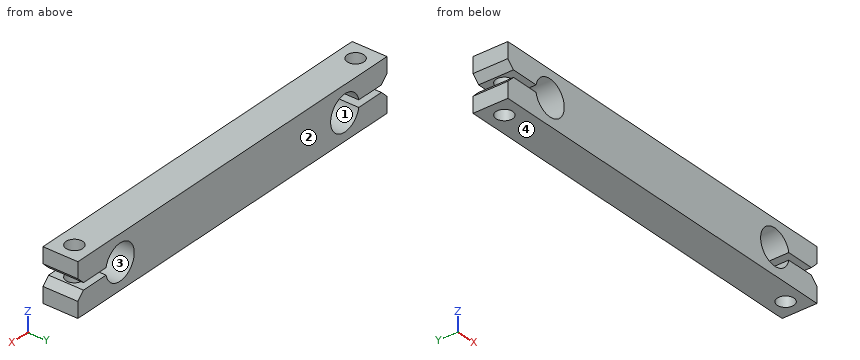
```python
from build123d import *

# Parameters (mm, degrees)
F0_W     = 34.925
F0_H     = 9.525
F0_R     = 3.2131
F1_DEPTH = 6.35
F2_R     = 1.524
F3_DEPTH = 9.525
F5_DEPTH = 6.351
F6_SIZE  = 1.27


with BuildPart() as f1:
    # F0 (on Front) → F1 (new body)
    with BuildSketch(Plane.XZ):
        with Locations((17.4625, 0)):
            Rectangle(F0_W, F0_H)
        with Locations((25.4, 0)):
            Circle(F0_R, mode=Mode.SUBTRACT)
    extrude(amount=F1_DEPTH)

    # F2 (on face) → F3 (cut, through all)
    with BuildSketch(Plane.XY.offset(4.7625)):
        with Locations((31.76905, -3.175)):
            Circle(F2_R)
    extrude(amount=-F3_DEPTH, mode=Mode.SUBTRACT)

    # F4 (on face) → F5 (cut, through all)
    with BuildSketch(Plane(origin=(0, 0, 0), x_dir=(-1, 0, 0), z_dir=(0, 1, 0))):
        with BuildLine():
            Line((-28.5497280216, 0.635), (-34.925, 0.635))
            Line((-34.925, 0.635), (-34.925, -0.635))
            Line((-34.925, -0.635), (-28.5497280216, -0.635))
            ThreePointArc((-28.5497280216, -0.635), (-28.6131, 0), (-28.5497280216, 0.635))
        make_face()
    extrude(amount=-F5_DEPTH, mode=Mode.SUBTRACT)

    # F6
    f6_edges = [f1.edges().sort_by_distance(p)[0] for p in [
        (34.925, -3.175, 0.635),
        (34.925, -3.175, -0.635),
    ]]
    chamfer(f6_edges, length=F6_SIZE)

    # F7: F1 across face


with BuildPart() as f1_1:
    add(f1.part)
    add(f1.part.mirror(Plane(origin=(0, -3.175, 0), x_dir=(0, -1, 0), z_dir=(-1, 0, 0))))


solid = f1_1.part
```
Build history of the part. All positions in model axes, mm. Face numbers are marked on the shaded views. Give positions to 0.01 mm unless a question says otherwise; leave off trailing zeros. Order: outer loops, then holes, each group sorted by start corner. A loop starts at its lowest first (then second) coordinate and runs counter-clockwise, first axis right, second up. Notation, with made-up numbers: M 56.25,69.25 L 81.25,69.25 A24 ccw 81.25,85.25 Z; hole C 68.5,-18.5 d10. An arc over 180 degrees is marked long. Write item = value, one per line. Start each with the question number.
(1) Two-plate mould, pull along Z, no slides. Class the marked faces 1, 2, 3 and 4: released by +Z, released by -Z, zero draft, split by the parting line, or undercut.
(2) Pin check, flat tip, straight feed: pin 1 Ø1.8 at (x, y) = (31.77, -3.18) entering from -Z. Stop position of the tip, or through.
(3) Slice it at A-A on x = -25.4. Write the cut outline in (y, z).
(4) Slice it at D-D on z = 0. Write the cut outline in (x, y), plus the area to 3 significant figures.
(5) Slice it at C-C on y = -0.75. Write the cut outline in (x, z) (1 decimal).
(6) Slice it at B-B on z = 2.5. Write the cut outline in (x, y) (3 decimals).
(7) Probe L1, parallel to Z at x = -29, y = -4 (1 decimal); L2, parallel to X at y = -3.5, z = 1.75; L3, parallel to X at y = -2.5, z = 2.5 (3 decimals). List the from-to ranges inside material, lowest first. Write a range as [from, to].
Responses:
q1.face_1 = undercut
q1.face_2 = zero draft
q1.face_3 = undercut
q1.face_4 = released by -Z
q2.pin_1 = through
q3.outline = M -6.35,-4.76 L 0,-4.76 L 0,-3.21 L -6.35,-3.21 Z; M -6.35,3.21 L 0,3.21 L 0,4.76 L -6.35,4.76 Z
q4.outline = M -22.19,-6.35 L 22.19,-6.35 L 22.19,0 L -22.19,0 Z
q4.area = 282 mm2
q5.outline = M -34.9,-4.8 L 34.9,-4.8 L 34.9,-1.9 L 33.7,-0.6 L 28.5,-0.6 A3.2 cw long 28.5,0.6 L 33.7,0.6 L 34.9,1.9 L 34.9,4.8 L -34.9,4.8 L -34.9,1.9 L -33.7,0.6 L -28.5,0.6 A3.2 cw long -28.5,-0.6 L -33.7,-0.6 L -34.9,-1.9 Z
q6.outline = M -34.925,-6.35 L -27.418,-6.35 L -27.418,0 L -34.925,0 Z; M -23.382,-6.35 L 23.382,-6.35 L 23.382,0 L -23.382,0 Z; M 27.418,-6.35 L 34.925,-6.35 L 34.925,0 L 27.418,0 Z; hole C -31.769,-3.175 d3.048; hole C 31.769,-3.175 d3.048
q7.L1 = [-4.8, -0.6], [0.6, 4.8]
q7.L2 = [-34.77, -33.26], [-30.28, -28.09], [-22.71, 22.71], [28.09, 30.28], [33.26, 34.77]
q7.L3 = [-34.925, -33.135], [-30.403, -27.418], [-23.382, 23.382], [27.418, 30.403], [33.135, 34.925]
